```python
from build123d import *

# Parameters (mm, degrees)
FILLET1_R = 2


with BuildPart() as part:
    # Sketch1 → Revolve5 (revolve)
    with BuildSketch(Plane.XY, mode=Mode.PRIVATE) as revolve5_sk:
        with BuildLine():
            ThreePointArc((7.653112519, 59), (0, 61.144988127), (-7.653112519, 59))
            Line((-7.653112519, 59), (-10, 59))
            Line((-10, 59), (-10, 66))
            Line((-10, 66), (10, 66))
            Line((10, 66), (10, 59))
            Line((10, 59), (7.653112519, 59))
        make_face()
    revolve(revolve5_sk.sketch.rotate(Axis((-1000, 0, 0), (1, 0, 0)), 90), axis=Axis((-1000, 0, 0), (1, 0, 0)))

    # Fillet1
    fillet1_edges = [part.edges().sort_by_distance(p)[0] for p in [
        (-7.653112519, 0, -59),
        (7.653112519, 0, -59),
    ]]
    fillet(fillet1_edges, radius=FILLET1_R)


solid = part.part
```
Verification items for the finished model (mm, model axes). Round coordinates to 2 decimals unless told otherwise and drop trailing zeros. Write each loop counter-clockwise with the first axis right and the second up, starting at its lowest first coordinate (ties: lowest second). Pieces come first, ordered by that corner, then holes. Notation, with made-up numbers: (-13, 61) - (19, 61) arc R9 ccw to (19, 75) - close; hole circle Ø3 at (57.25, -6.5). An arc over 180 degrees is marked (long way). Answer as a JSON object with one key per item and string values. Group by question number.
Q1. Thickness scan on line 1 (Y direction, x = 9, z = 0); line 2 (Y direction, x = 1.5, z = -12.5); line 3 (Z direction, x = -5, y = 15.5). Record the ranges inside material, lowest first.
Q2. Go/stop test with flat-tipped pins: pin 1 Ø1 at (x, y) = (5, -33.5) entering from -Z; pin 2 Ø3 at (x, y) = (-7, -14.5) entering from -Z; pin 3 Ø3 at (x, y) = (1.5, 25.5) entering from +Z. Record where each tip stops, or that it passes through.
Q3. Section check A-A, the plane x = 2.5. Enter the section's corners in (y, z), plus the area to 3 significant figures.
Q4. Mould release check, pull along Y, two halves, no side actions. Record for faces 1 (the cylindrical face through (0.14, -19.825, 62.952)), 2 (the cylindrical face through (-9.11, -17.722, 56.275)), 3 (the flat face through (-10, 34, 49)): released by +Y, released by -Y, zero draft, split by the parting line, or undercut.
Q5. Section check B-B, the plane x = -4.75. Enter the section's corners in (y, z), plus the area to 3 significant figures.
Found:
{
 "1": {"line 1": "y = -66 to -59, 59 to 66", "line 2": "y = -64.81 to -59.78, 59.78 to 64.81", "line 3": "z = -64.15 to -58.24, 58.24 to 64.15"},
 "2": {"pin 1": "stops at z = -57.16", "pin 2": "stops at z = -64.71", "pin 3": "stops at z = 61.48"},
 "3": {"outline": "circle Ø132 at (0, 0); hole circle Ø121.86 at (0, 0)", "area": "2,020 mm^2"},
 "4": {"face 1": "split by the parting line", "face 2": "undercut", "face 3": "zero draft"},
 "5": {"outline": "circle Ø132 at (0, 0); hole circle Ø120.72 at (0, 0)", "area": "2,240 mm^2"}
}
